Part model, mm, in its own coordinate system. Face numbers are marked on the shaded views. A direction names the side the tool comes from. Give positions to 0.01 mm unless a question says otherwise; leave off trailing zeros. Loops run counter-clockwise (first coordinate to the right, second up) from the corner with the lowest first, then second, coordinate; pieces in that order, holes last. Notation, with made-up numbers: M 88,50 L 120,50 A12 cw 120,59 Z; hole C -16,40 d3. An arc over 180 degrees is marked long. Answer in a Markdown table with one row per item.
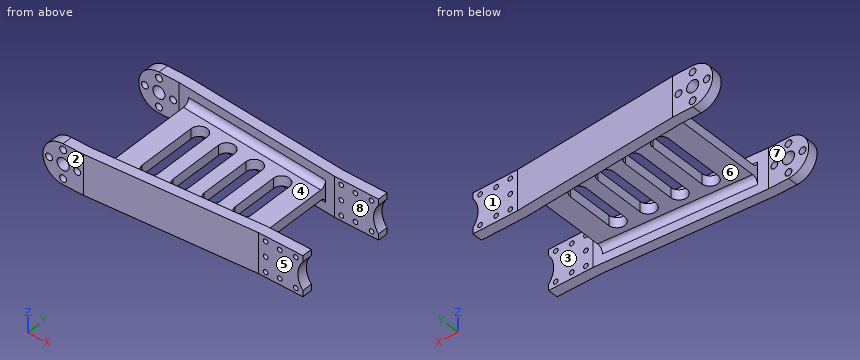
from build123d import *

# Parameters (mm, degrees)
SKETCH_1_R           = 10
SKETCH_1_R_2         = 3
SKETCH_1_R_3         = 1.7
SKETCH_1_R_4         = 1.15
EXTRUDE_1_DEPTH      = 11
EXTRUDE_START        = 51
SKETCH_1_3_R         = 1.15
SKETCH_1_3_R_2       = 10
SKETCH_1_3_R_3       = 3
SKETCH_1_3_R_4       = 1.7
EXTRUDE_2_DEPTH      = 11
SKETCH_4_W           = 10
SKETCH_4_H           = 46
SKETCH_4_H_2         = 6
SKETCH_4_W_2         = 22
SKETCH_4_H_3         = 40
CUT_EXTRUDE_1_DEPTH  = 132.301180497
EXTRUDE_4_DEPTH      = 2.5
EXTRUDE_4_DEPTH_BACK = 2.5
CUT_EXTRUDE_2_DEPTH  = 131.369666717
FILLET_1_R           = 3


with BuildPart() as part:
    # Sketch 1 → Extrude 1 (new body)
    # profile 1 of 2: a face of its own
    with BuildSketch(Plane(origin=(0, 0, 0), x_dir=(1, 0, 0), z_dir=(0, 1, 0))):
        Circle(SKETCH_1_R)
        with Locations(Location((0, 0, 0), (0, 0, 270))):
            Circle(SKETCH_1_R_2, mode=Mode.SUBTRACT)
        with Locations(Location((-7, 0, 0), (0, 0, 270))):
            Circle(SKETCH_1_R_3, mode=Mode.SUBTRACT)
        with Locations(Location((0, -7, 0), (0, 0, 270))):
            Circle(SKETCH_1_R_3, mode=Mode.SUBTRACT)
        with Locations(Location((7, 0, 0), (0, 0, 270))):
            Circle(SKETCH_1_R_3, mode=Mode.SUBTRACT)
        with Locations(Location((0, 7, 0), (0, 0, 270))):
            Circle(SKETCH_1_R_3, mode=Mode.SUBTRACT)
    # profile 2 of 2: a face of its own
    with BuildSketch(Plane(origin=(0, 0, 0), x_dir=(1, 0, 0), z_dir=(0, 1, 0))):
        with BuildLine():
            Line((114, 10), (0, 10))
            ThreePointArc((0, 10), (7.071067812, 7.071067812), (10, 0))
            ThreePointArc((10, 0), (7.071067812, -7.071067812), (0, -10))
            Line((0, -10), (114, -10))
            Line((114, -10), (114, -6.982120022))
            ThreePointArc((114, -6.982120022), (111.5, 0), (114, 6.982120022))
            Line((114, 6.982120022), (114, 10))
        make_face()
        with Locations(Location((95.5, -7.5, 0), (0, 0, 270))):
            Circle(SKETCH_1_R_4, mode=Mode.SUBTRACT)
        with Locations(Location((102.5, -7, 0), (0, 0, 270))):
            Circle(SKETCH_1_R_4, mode=Mode.SUBTRACT)
        with Locations(Location((110.5, -7.5, 0), (0, 0, 270))):
            Circle(SKETCH_1_R_4, mode=Mode.SUBTRACT)
        with Locations(Location((95.5, 0, 0), (0, 0, 270))):
            Circle(SKETCH_1_R_4, mode=Mode.SUBTRACT)
        with Locations(Location((95.5, 7.5, 0), (0, 0, 270))):
            Circle(SKETCH_1_R_4, mode=Mode.SUBTRACT)
        with Locations(Location((102.5, 7, 0), (0, 0, 270))):
            Circle(SKETCH_1_R_4, mode=Mode.SUBTRACT)
        with Locations(Location((110.5, 7.5, 0), (0, 0, 270))):
            Circle(SKETCH_1_R_4, mode=Mode.SUBTRACT)
    extrude(amount=EXTRUDE_1_DEPTH)


with BuildPart() as body_2:
    # Sketch 1_3 → Extrude 2 (new body)
    # profile 1 of 2: a face of its own
    with BuildSketch(Plane(origin=(0, 0, 0), x_dir=(1, 0, 0), z_dir=(0, 1, 0)).offset(EXTRUDE_START)):
        with BuildLine():
            Line((114, 10), (0, 10))
            ThreePointArc((0, 10), (7.071067812, 7.071067812), (10, 0))
            ThreePointArc((10, 0), (7.071067812, -7.071067812), (0, -10))
            Line((0, -10), (114, -10))
            Line((114, -10), (114, -6.982120022))
            ThreePointArc((114, -6.982120022), (111.5, 0), (114, 6.982120022))
            Line((114, 6.982120022), (114, 10))
        make_face()
        with Locations(Location((95.5, -7.5, 0), (0, 0, 270))):
            Circle(SKETCH_1_3_R, mode=Mode.SUBTRACT)
        with Locations(Location((102.5, -7, 0), (0, 0, 270))):
            Circle(SKETCH_1_3_R, mode=Mode.SUBTRACT)
        with Locations(Location((110.5, -7.5, 0), (0, 0, 270))):
            Circle(SKETCH_1_3_R, mode=Mode.SUBTRACT)
        with Locations(Location((95.5, 0, 0), (0, 0, 270))):
            Circle(SKETCH_1_3_R, mode=Mode.SUBTRACT)
        with Locations(Location((95.5, 7.5, 0), (0, 0, 270))):
            Circle(SKETCH_1_3_R, mode=Mode.SUBTRACT)
        with Locations(Location((102.5, 7, 0), (0, 0, 270))):
            Circle(SKETCH_1_3_R, mode=Mode.SUBTRACT)
        with Locations(Location((110.5, 7.5, 0), (0, 0, 270))):
            Circle(SKETCH_1_3_R, mode=Mode.SUBTRACT)
    # profile 2 of 2: a face of its own
    with BuildSketch(Plane(origin=(0, 0, 0), x_dir=(1, 0, 0), z_dir=(0, 1, 0)).offset(EXTRUDE_START)):
        Circle(SKETCH_1_3_R_2)
        with Locations(Location((0, 0, 0), (0, 0, 270))):
            Circle(SKETCH_1_3_R_3, mode=Mode.SUBTRACT)
        with Locations(Location((-7, 0, 0), (0, 0, 270))):
            Circle(SKETCH_1_3_R_4, mode=Mode.SUBTRACT)
        with Locations(Location((0, -7, 0), (0, 0, 270))):
            Circle(SKETCH_1_3_R_4, mode=Mode.SUBTRACT)
        with Locations(Location((7, 0, 0), (0, 0, 270))):
            Circle(SKETCH_1_3_R_4, mode=Mode.SUBTRACT)
        with Locations(Location((0, 7, 0), (0, 0, 270))):
            Circle(SKETCH_1_3_R_4, mode=Mode.SUBTRACT)
    extrude(amount=EXTRUDE_2_DEPTH)


with BuildPart() as cut_extrude_1_tool:
    # Sketch 4 → Cut-Extrude 1 (new, through all)
    with BuildSketch(Plane.XY.offset(10)):
        with Locations((5, 28)):
            Rectangle(SKETCH_4_W, SKETCH_4_H)
        with Locations((5, 54)):
            Rectangle(SKETCH_4_W, SKETCH_4_H_2)
        Polygon((-10, 5), (0, 5), (0, 51), (0, 57), (-10, 57), align=None)
        with Locations((103, 31)):
            Rectangle(SKETCH_4_W_2, SKETCH_4_H_3)
        Polygon((10, 51), (10, 5), (92, 11), (92, 51), align=None)
        Polygon((10, 57), (10, 51), (92, 51), align=None)
        Polygon((114, 6), (92, 6), (10, 0), (114, 0), align=None)
        Polygon((114, 62), (10, 62), (92, 56), (114, 56), align=None)
    extrude(amount=-CUT_EXTRUDE_1_DEPTH)


with BuildPart() as part_1:
    add(part.part)

    # Cut-Extrude 1: cut by cut_extrude_1_tool
    add(cut_extrude_1_tool.part, mode=Mode.SUBTRACT)



with BuildPart() as body_2_1:
    add(body_2.part)

    # Cut-Extrude 1: cut by cut_extrude_1_tool
    add(cut_extrude_1_tool.part, mode=Mode.SUBTRACT)


with BuildPart() as part_2:
    add(part_1.part)

    add(body_2_1.part)  # Extrude 4 merges body 2
    # Sketch 5 → Extrude 4 (add, two sides: drawn at the far end of the back side and taken through both)
    with BuildSketch(Plane.XY.offset(-EXTRUDE_4_DEPTH_BACK)):
        Polygon((15, 56.634146341), (15, 5.365853659), (87.5, 10.670731707), (87.5, 51.329268293), align=None)
    extrude(amount=EXTRUDE_4_DEPTH + EXTRUDE_4_DEPTH_BACK)

    # Sketch 9 → Cut-Extrude 2 (cut, through all)
    with BuildSketch(Plane.XY.offset(2.5)):
        with BuildLine():
            Line((33.5, 45.573170732), (33.5, 16.426829268))
            ThreePointArc((33.5, 16.426829268), (29.5, 12.426829268), (25.5, 16.426829268))
            Line((25.5, 16.426829268), (25.5, 45.573170732))
            ThreePointArc((25.5, 45.573170732), (29.5, 49.573170732), (33.5, 45.573170732))
        make_face()
        with BuildLine():
            Line((48, 44.512195122), (48, 17.487804878))
            ThreePointArc((48, 17.487804878), (44, 13.487804878), (40, 17.487804878))
            Line((40, 17.487804878), (40, 44.512195122))
            ThreePointArc((40, 44.512195122), (44, 48.512195122), (48, 44.512195122))
        make_face()
        with BuildLine():
            Line((62.5, 43.451219512), (62.5, 18.548780488))
            ThreePointArc((62.5, 18.548780488), (58.5, 14.548780488), (54.5, 18.548780488))
            Line((54.5, 18.548780488), (54.5, 43.451219512))
            ThreePointArc((54.5, 43.451219512), (58.5, 47.451219512), (62.5, 43.451219512))
        make_face()
        with BuildLine():
            Line((77, 42.390243902), (77, 19.609756098))
            ThreePointArc((77, 19.609756098), (73, 15.609756098), (69, 19.609756098))
            Line((69, 19.609756098), (69, 42.390243902))
            ThreePointArc((69, 42.390243902), (73, 46.390243902), (77, 42.390243902))
        make_face()
    extrude(amount=-CUT_EXTRUDE_2_DEPTH, mode=Mode.SUBTRACT)

    # Fillet 1
    fillet_1_edges = [part_2.edges().sort_by_distance(p)[0] for p in [
        (51.25, 53.981707317, -2.5),
        (51.25, 8.018292683, -2.5),
        (51.25, 53.981707317, 2.5),
        (51.25, 8.018292683, 2.5),
    ]]
    fillet(fillet_1_edges, radius=FILLET_1_R)


solid = part_2.part
(1) Pull direction Y, two halves, no side cores. Call the marked faces 1, 2 and 3: +Y half, -Y half, draft (parallel to the pull), parting line (faces both ways), or undercut.
Recorded:
| item | result |
|---|---|
| face 1 | +Y half |
| face 2 | -Y half |
| face 3 | undercut |
(2) Drill centre lines: line 1 along X through (y, z) = (30.5, 0.25); line 2 along Z through (x, y) = (0, 59.45); line 3 along Y through (x, z) = (-3.5, 0.5). Where is each one in solid material? Low to high.
Recorded:
| item | result |
|---|---|
| line 1 | x = 15 to 25.5, 33.5 to 40, 48 to 54.5, 62.5 to 69, 77 to 87.5 |
| line 2 | z = -10 to -8.7, -5.3 to -3, 3 to 5.3, 8.7 to 10 |
| line 3 | y = 0 to 5, 57 to 62 |
(3) Saw through at B-B (y = 29). Write the cut outline in (x, z), plus the area to 4 significant figures.
Recorded:
| item | result |
|---|---|
| outline | M 15,-2.5 L 25.5,-2.5 L 25.5,2.5 L 15,2.5 Z; M 33.5,-2.5 L 40,-2.5 L 40,2.5 L 33.5,2.5 Z; M 48,-2.5 L 54.5,-2.5 L 54.5,2.5 L 48,2.5 Z; M 62.5,-2.5 L 69,-2.5 L 69,2.5 L 62.5,2.5 Z; M 77,-2.5 L 87.5,-2.5 L 87.5,2.5 L 77,2.5 Z |
| area | 202.5 mm^2 |
(4) Which spindle directions (+Z, -Z, +X, -X, +Y, -Y) get a long thin tool onto all of the face, cutting with end or side? Do the marked faces 4, 5, 6, 7 and 8. Say none if no direction does.
Recorded:
| item | result |
|---|---|
| face 4 | +Z, -X |
| face 5 | +Z, -Z, +X, -Y |
| face 6 | -Z, -X |
| face 7 | +Z, -Z, -X |
| face 8 | +Z, -Z, +X |
(5) Pin check, flat tips, straight feed: pin 1 Ø3 at (x, z) = (100.5, 8) entering from -Y; pin 2 Ø5.5 at (y, z) = (35.5, 0) entering from +X; pin 3 Ø5.5 at (x, z) = (0, -7) entering from +Y; pin 4 Ø3 at (x, z) = (110.5, 7.5) entering from +Y. Stop position of each tip, or through.
Recorded:
| item | result |
|---|---|
| pin 1 | stops at y = 6 |
| pin 2 | stops at x = 87.5 |
| pin 3 | stops at y = 62 |
| pin 4 | stops at y = 56 |
(6) Saw through at A-A (x = 7). Write the cut outline in (y, z).
Recorded:
| item | result |
|---|---|
| outline | M 0,-10 L 5,-10 L 5,-1.7 L 0,-1.7 Z; M 0,1.7 L 5,1.7 L 5,10 L 0,10 Z; M 57,-10 L 62,-10 L 62,-1.7 L 57,-1.7 Z; M 57,1.7 L 62,1.7 L 62,10 L 57,10 Z |
